The drawing under review shows one solid part. Ordinate dimensions are in mm from its lowest x, y, z. Round coordinates to 2 decimals unless told otherwise and drop trailing zeros. Order: outer loops, then holes, each group sorted by start corner. A loop starts at its lowest first (then second) coordinate and runs counter-clockwise, first axis right, second up. Notation, with made-up numbers: M 70.5,76 L 122.5,76 A27 ccw 122.5,102 Z; hole C 61.25,-36 d8. An arc over 180 degrees is marked long. Use a Markdown table: item, result.
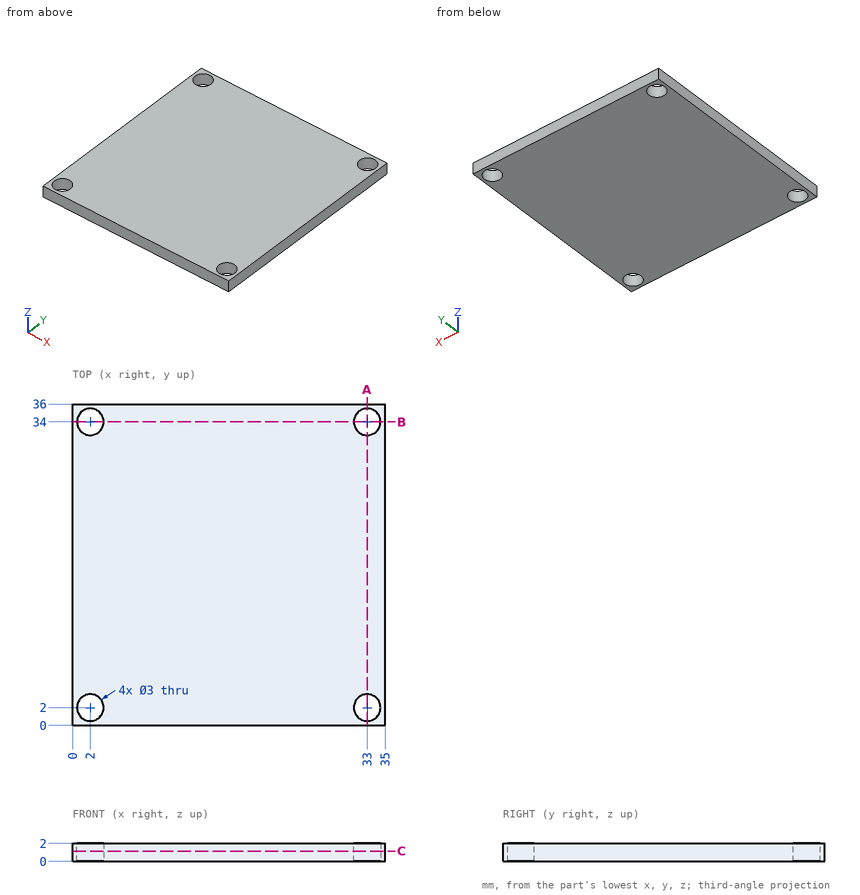
Q1. Clearance check with a flat-ended pin moving along its axis: pin 1 (4 mm diameter, centred on x = 2, y = 2, fed in from +Z). State where the tip first meets the part, or that it passes through.
Determined:
| item | result |
|---|---|
| pin 1 | stops at z = 2 |
Q2. Add section A-A (x = 33). Write out the cut boundary in (y, z), then the cut area to 3 significant figures.
Determined:
| item | result |
|---|---|
| outline | M 0,0 L 0.5,0 L 0.5,2 L 0,2 Z; M 3.5,0 L 32.5,0 L 32.5,2 L 3.5,2 Z; M 35.5,0 L 36,0 L 36,2 L 35.5,2 Z |
| area | 60.0 mm^2 |
Q3. Add section B-B (y = 34). Write out the cut boundary in (x, z).
Determined:
| item | result |
|---|---|
| outline | M 0,0 L 0.5,0 L 0.5,2 L 0,2 Z; M 3.5,0 L 31.5,0 L 31.5,2 L 3.5,2 Z; M 34.5,0 L 35,0 L 35,2 L 34.5,2 Z |
Q4. Add section C-C (z = 1.15). Write out the cut boundary in (x, y), then the cut area to 3 significant figures.
Determined:
| item | result |
|---|---|
| outline | M 0,0 L 35,0 L 35,36 L 0,36 Z; hole C 2,2 d3; hole C 2,34 d3; hole C 33,2 d3; hole C 33,34 d3 |
| area | 1,230 mm^2 |
Q5. Wall thickness on line 1 along Y through (x, z) = (33, 1.3): over which ranges is the line inside the solid? List them lowest first. Write a range as [from, to].
Determined:
| item | result |
|---|---|
| line 1 | y = [0, 0.5], [3.5, 32.5], [35.5, 36] |
